Input: part model. Units: mm. Frame: model coordinates. Face numbers are marked on the shaded views. Coordinates: 2 decimals unless noted, no trailing zeros. Order: outer loops, then holes, each group sorted by start corner. A loop starts at its lowest first (then second) coordinate and runs counter-clockwise, first axis right, second up. Notation, with made-up numbers: (80.25, -13.75) - (137.25, -13.75) arc R25 ccw to (137.25, 20.25) - close; hole circle Ø11 at (42, 86). An arc over 180 degrees is marked (long way). Answer as CSV lines item,"result". Start each with the question number.
Item 1: Section A-A (x = 0). Output: boundary loops of the cut face in (y, z) (3 decimals), and give its area (3 significant figures).
Item 2: Draft query along Y for the marked faces 1, 2 and 3. Return one class per face: +Y half, -Y half, draft (parallel to the pull), parting line (faces both ways), or undercut.
Item 3: Material intervals for line 1 along Z through (x, y) = (-6.5, -21.5); line 2 along Y through (x, z) = (-14, 7.9); line 3 along Y through (x, z) = (0, 8.7), sorted ascending.
Item 4: First-contact query: pin 1 (3 mm diameter, centred on x = 6.5, z = 7, fed in from +Y); pin 2 (4 mm diameter, centred on x = 17, y = -8.5, fed in from +Z); pin 3 (2 mm diameter, centred on y = -2.5, z = 6, fed in from +X). Flat tips, straight axial feed; report the tip coordinate or a pass-through.
Item 5: Section C-C (z = 6.1). Output: boundary loops of the cut face in (x, y), and give its area (3 significant figures).
from build123d import *


with BuildPart() as f2:
    # F0 (on Front) → F2 (revolve)
    with BuildSketch(Plane.XZ):
        with BuildLine():
            Line((27.305, 7.601389), (0, 7.601389))
            Line((0, 7.601389), (0, 4.483546))
            Line((0, 4.483546), (29.317615, 4.483546))
            ThreePointArc((29.317615, 4.483546), (30.046057, 4.713222), (30.511025, 5.31918))
            Line((30.511025, 5.31918), (31.814121, 8.899409))
            ThreePointArc((31.814121, 8.899409), (31.752887, 9.364532), (31.336757, 9.581155))
            Line((31.336757, 9.581155), (28.615081, 9.581155))
            ThreePointArc((28.615081, 9.581155), (28.30583, 9.476179), (28.124391, 9.204635))
            Line((28.124391, 9.204635), (27.79569, 7.977909))
            ThreePointArc((27.79569, 7.977909), (27.614251, 7.706366), (27.305, 7.601389))
        make_face()
    revolve(axis=Axis((0, 0, 5.026823), (0, 0, -1)))


solid = f2.part
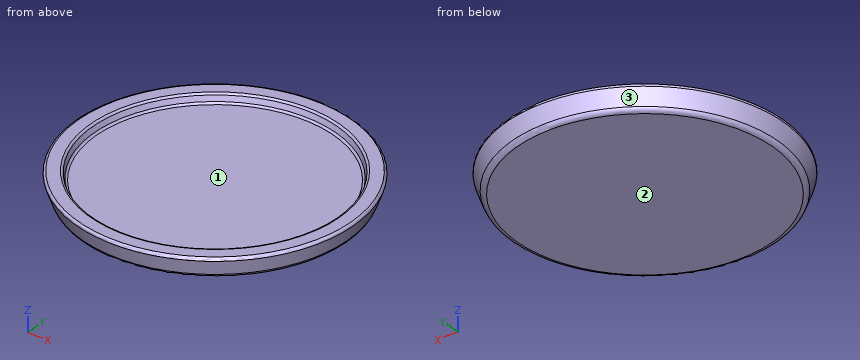
Determined:
1,outline,"(-31.814, 8.899) - (-30.511, 5.319) arc R1.27 ccw to (-29.318, 4.484) - (29.318, 4.484) arc R1.27 ccw to (30.511, 5.319) - (31.814, 8.899) arc R0.508 ccw to (31.337, 9.581) - (28.615, 9.581) arc R0.508 ccw to (28.124, 9.205) - (27.796, 7.978) arc R0.508 cw to (27.305, 7.601) - (-27.305, 7.601) arc R0.508 cw to (-27.796, 7.978) - (-28.124, 9.205) arc R0.508 ccw to (-28.615, 9.581) - (-31.337, 9.581) arc R0.508 ccw to start"
1,area,"206 mm^2"
2,face 1,"undercut"
2,face 2,"draft"
2,face 3,"parting line"
3,line 1,"z = 4.48 to 7.6"
3,line 2,"y = -28.16 to -23.98, 23.98 to 28.16"
3,line 3,"y = -31.74 to -27.99, 27.99 to 31.74"
4,pin 1,"stops at y = 31.07"
4,pin 2,"stops at z = 7.6"
4,pin 3,"stops at x = 31.03"
5,outline,"circle Ø61.59 at (0, 0)"
5,area,"2,980 mm^2"
